Build history of the part. All positions in model axes, mm. Face numbers are marked on the shaded views. Round coordinates to 2 decimals unless told otherwise and drop trailing zeros. Loops run counter-clockwise (first coordinate to the right, second up) from the corner with the lowest first, then second, coordinate; pieces in that order, holes last.
from build123d import *

# Parameters (mm, degrees)
F1_DEPTH = 12.7


with BuildPart() as f1:
    # F0 (on Right) → F1 (new body)
    with BuildSketch(Plane.YZ):
        with BuildLine():
            Line((-47.625, 88.9), (-73.025, 88.9))
            ThreePointArc((-73.025, 88.9), (-88.740448, 82.390448), (-95.25, 66.675))
            Line((-95.25, 66.675), (-95.25, 6.35))
            Line((-95.25, 6.35), (95.25, 6.35))
            Line((95.25, 6.35), (95.25, 66.675))
            ThreePointArc((95.25, 66.675), (88.740448, 82.390448), (73.025, 88.9))
            Line((73.025, 88.9), (47.625, 88.9))
            ThreePointArc((47.625, 88.9), (31.909552, 82.390448), (25.4, 66.675))
            Line((25.4, 66.675), (25.4, 70.083901))
            ThreePointArc((25.4, 70.083901), (18.890448, 54.368453), (3.175, 47.858901))
            Line((3.175, 47.858901), (-3.175, 47.858901))
            ThreePointArc((-3.175, 47.858901), (-18.890448, 54.368453), (-25.4, 70.083901))
            Line((-25.4, 70.083901), (-25.4, 66.675))
            ThreePointArc((-25.4, 66.675), (-31.909552, 82.390448), (-47.625, 88.9))
        make_face()
    extrude(amount=F1_DEPTH)


solid = f1.part
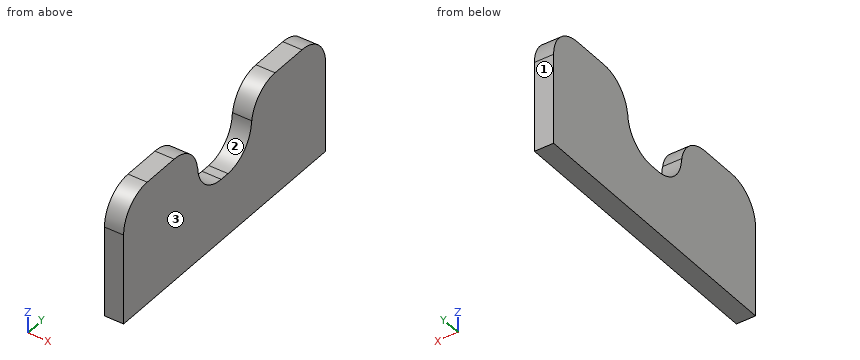
(1) Probe line 1 (Y direction, x = 8.5, z = 84); line 2 (Y direction, x = 7.5, z = 77); line 3 (Z direction, x = 4, y = 17). List the from-to ranges inside material, lowest first.
Responses:
line 1: y = -86.95 to -33.7, 33.7 to 86.95
line 2: y = -92.71 to -27.94, 27.94 to 92.71
line 3: z = 6.35 to 52.68
(2) Slice it at C-C on y = 33. List the corners of the cut face in (x, z).
Responses:
outline: (0, 6.35) - (12.7, 6.35) - (12.7, 83.41) - (0, 83.41) - close
(3) Pin check, flat tips, straight feed: P1, Ø3, axis at x = 7, y = -1, coming from the +Z side; P2, Ø1.7, axis at x = 7, z = 68.5, coming from the +Y side; P3, Ø6, axis at y = -56.5, z = 31.5, coming from the -X side; P4, Ø2.5, axis at x = 8, z = 69, coming from the -Y side. Stop position of each tip, or through.
Responses:
P1: stops at z = 47.86
P2: stops at y = 95.23
P3: stops at x = 0
P4: stops at y = -95.22
(4) Slice it at A-A on x = 8. List the corners of the cut face in (y, z) (3 decimals), plus the area to 3 significant figures.
Responses:
outline: (-95.25, 6.35) - (95.25, 6.35) - (95.25, 66.675) arc R22.225 ccw to (73.025, 88.9) - (47.625, 88.9) arc R22.225 ccw to (25.4, 66.675) - (25.4, 70.084) arc R22.225 cw to (3.175, 47.859) - (-3.175, 47.859) arc R22.225 cw to (-25.4, 70.084) - (-25.4, 66.675) arc R22.225 ccw to (-47.625, 88.9) - (-73.025, 88.9) arc R22.225 ccw to (-95.25, 66.675) - close
area: 13,400 mm2
(5) Slice it at D-D on z = 59. List the corners of the cut face in (x, y).
Responses:
outline: (0, -95.25) - (12.7, -95.25) - (12.7, -22.44) - (0, -22.44) - close; (0, 22.44) - (12.7, 22.44) - (12.7, 95.25) - (0, 95.25) - close
(6) Pull direction Y, two halves, no side cores. Call the marked faces 1, 2 and 3: +Y half, -Y half, draft (parallel to the pull), parting line (faces both ways), or undercut.
Responses:
face 1: +Y half
face 2: undercut
face 3: draft
(7) Slice it at B-B on z = 78. List the corners of the cut face in (x, y), plus the area to 3 significant figures.
Responses:
outline: (0, -92.15) - (12.7, -92.15) - (12.7, -28.5) - (0, -28.5) - close; (0, 28.5) - (12.7, 28.5) - (12.7, 92.15) - (0, 92.15) - close
area: 1,620 mm2
